Build history of the part. All positions in model axes, mm. A direction names the side the tool comes from. Round coordinates to 2 decimals unless told otherwise and drop trailing zeros. Write each loop counter-clockwise with the first axis right and the second up, starting at its lowest first coordinate (ties: lowest second). Pieces come first, ordered by that corner, then holes. Notation, with made-up numbers: (-5, -11.5) -> (35, -11.5) arc R18 cw to (35, -7.5) -> close; hole circle Ø7 at (34.5, 4). An arc over 180 degrees is marked (long way). Answer in a Markdown table with one row per item.
```python
from build123d import *

# Parameters (mm, degrees)
F0_W     = 39.285619
F0_H     = 56.238633
F1_DEPTH = 25.4
F2_R     = 9.880036
F3_DEPTH = 12.7
F5_R     = 7.52441
F6_DEPTH = 38.101


with BuildPart() as f1:
    # F0 (on Front) → F1 (new body)
    with BuildSketch(Plane.XZ):
        with Locations((-9.948956, 21.362619)):
            Rectangle(F0_W, F0_H)
    extrude(amount=F1_DEPTH)

    # F2 (on face) → F3 (join)
    with BuildSketch(Plane.XZ.offset(25.4)):
        with Locations((-10.390805, 20.258)):
            Circle(F2_R)
    extrude(amount=F3_DEPTH)

    # F5 (on face) → F6 (cut, through all)
    with BuildSketch(Plane.XZ.offset(38.1)):
        with Locations((-10.390805, 20.478925)):
            Circle(F5_R)
    extrude(amount=-F6_DEPTH, mode=Mode.SUBTRACT)


solid = f1.part
```
Q1. Two-plate mould, pull along Z, no slides. Class faces 3 (the cylindrical face through (-11.37, -19.32, 27.94)), 4 (the flat face through (-6, 0, 28)), 5 (the flat face through (-10, -13, 49.482)): released by +Z, released by -Z, zero draft, split by the parting line, or undercut.
A:
| item | result |
|---|---|
| face 3 | undercut |
| face 4 | zero draft |
| face 5 | released by +Z |
Q2. Wall check: line 1 (X direction, y = -5.5, z = 20); line 2 (Y direction, x = -22, z = 47.5); line 3 (X direction, y = -32, z = 15). Give the ranges that are in metal, low to high. Write a range as [from, to].
A:
| item | result |
|---|---|
| line 1 | [-29.59, -17.9], [-2.88, 9.69] |
| line 2 | [-25.4, 0] |
| line 3 | [-18.76, -15.55], [-5.23, -2.03] |
Q3. Saw through at D-D on x = 3. Write the cut outline in (y, z), plus the area to 3 significant figures.
A:
| item | result |
|---|---|
| outline | (-25.4, -6.76) -> (0, -6.76) -> (0, 49.48) -> (-25.4, 49.48) -> close |
| area | 1,430 mm² |
Q4. Drop flat-ended pins along their axis: P1, Ø4, axis at y = -29.5, z = 13.5, coming from the -X side; P2, Ø1.5, axis at x = -15, z = 39, coming from the -Y side. Give the stop position or say it passes through.
A:
| item | result |
|---|---|
| P1 | x = -19.05 |
| P2 | y = -25.4 |
Q5. Saw through at C-C on y = -2.5. Write the cut outline in (x, z), plus the area to 3 significant figures.
A:
| item | result |
|---|---|
| outline | (-29.59, -6.76) -> (9.69, -6.76) -> (9.69, 49.48) -> (-29.59, 49.48) -> close; hole circle Ø15.05 at (-10.39, 20.48) |
| area | 2,030 mm² |
Q6. Saw through at A-A on z = 16. Write the cut outline in (x, y), plus the area to 3 significant figures.
A:
| item | result |
|---|---|
| outline | (-29.59, -25.4) -> (-19.31, -25.4) -> (-19.31, -38.1) -> (-16.44, -38.1) -> (-16.44, 0) -> (-29.59, 0) -> close; (-4.34, -38.1) -> (-1.48, -38.1) -> (-1.48, -25.4) -> (9.69, -25.4) -> (9.69, 0) -> (-4.34, 0) -> close |
| area | 764 mm² |
Q7. Which spindle directions (+Z, -Z, +X, -X, +Y, -Y) get a long thin tool onto all of the face, cutting with end or side? Do faces 1 (the flat face through (-29.592, -13, 21)), 2 (the cylindrical face through (-18.231, -31.661, 14.246)). Say none if no direction does.
A:
| item | result |
|---|---|
| face 1 | +Z, -Z, -X, +Y, -Y |
| face 2 | -Y |
Q8. Saw through at B-B on x = -14. Write the cut outline in (y, z).
A:
| item | result |
|---|---|
| outline | (-38.1, 11.06) -> (-25.4, 11.06) -> (-25.4, -6.76) -> (0, -6.76) -> (0, 13.88) -> (-38.1, 13.88) -> close; (-38.1, 27.08) -> (0, 27.08) -> (0, 49.48) -> (-25.4, 49.48) -> (-25.4, 29.46) -> (-38.1, 29.46) -> close |
